Verification items for this drawing (mm, ordinates from the low corner). A direction names the side the tool comes from. Round coordinates to 2 decimals unless told otherwise and drop trailing zeros. Write each loop counter-clockwise with the first axis right and the second up, starting at its lowest first coordinate (ties: lowest second). Pieces come first, ordered by that corner, then holes.
Item 1: Access from +Z, -Z, +X, -X, +Y, -Y to the whole of each face (thin tool, end or side, straight path). Record for the marked faces 1 and 2.
Item 2: Cross-section at B-B (x = 8.5). Enter the section's corners in (y, z).
Item 3: Depth check by flat-ended pin: P1, Ø3.5, axis at x = 61, z = 4, coming from the +Y side. Enter the tip coordinate at first touch or a pass-through.
Item 4: Cross-section at A-A (z = 3). Enter the section's corners in (x, y), then the cut area to 4 significant figures.
Item 5: Scan lines: probe 1 along Z at (x, y) = (13, 3.25); probe 2 along X at (y, z) = (4, 5.3); probe 3 along Y at (x, z) = (8, 5.6). Record each from-to range of solid material in increasing order.
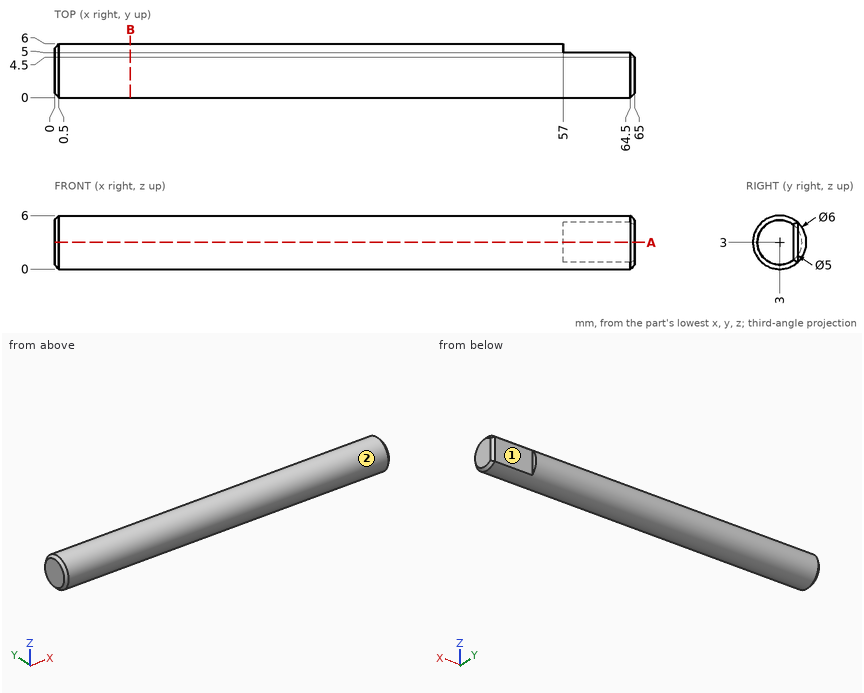
Resolved:
1. face 1: +Z, -Z, +X, +Y
1. face 2: +X, -X
2. outline: circle Ø6 at (3, 3)
3. P1: stops at y = 5
4. outline: (0, 0.5) - (0.5, 0) - (64.5, 0) - (65, 0.5) - (65, 4.5) - (64.5, 5) - (57, 5) - (57, 6) - (0.5, 6) - (0, 5.5) - close
4. area: 381.5 mm2
5. probe 1: z = 0.01 to 5.99
5. probe 2: x = 0.01 to 64.99
5. probe 3: y = 1.5 to 4.5
